Here's the drawing with two shaded views (mm, measured from the low corner). I have some questions. Round coordinates to 2 decimals unless told otherwise and drop trailing zeros. Loops run counter-clockwise (first coordinate to the right, second up) from the corner with the lowest first, then second, coordinate; pieces in that order, holes last.
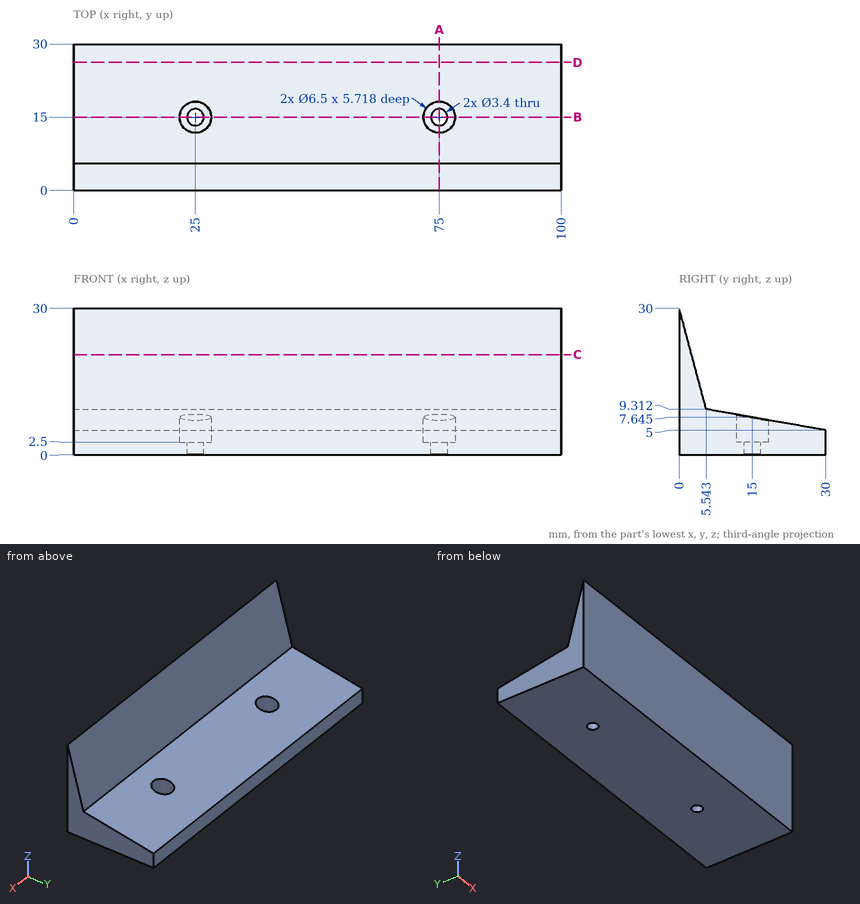
(1) If we section it at B-B, the plane y = 15: State how many separate pieces and enclosed holes the cut face has.
Worked answers:
separate pieces: 3
enclosed holes: 0
(2) If we section it at C-C, the plane z = 20.5: List the corners of the cut face in (x, y) for me (1 decimal).
Worked answers:
outline: (0, 0) - (100, 0) - (100, 2.5) - (0, 2.5) - close
(3) If we section it at D-D, the plane y = 26.25: List the corners of the cut face in (x, z) for me.
Worked answers:
outline: (0, 0) - (100, 0) - (100, 5.66) - (0, 5.66) - close
(4) If we section it at A-A, the plane x = 75: List the corners of the cut face in (y, z) for me.
Worked answers:
outline: (0, 0) - (13.3, 0) - (13.3, 2.5) - (11.75, 2.5) - (11.75, 8.22) - (5.54, 9.31) - (0, 30) - close; (16.7, 0) - (30, 0) - (30, 5) - (18.25, 7.07) - (18.25, 2.5) - (16.7, 2.5) - close
(5) Will these pins go through, and if not, where does the flat tip stop? P1, Ø10, axis at x = 51.5, y = 19, coming from the -Z side; P2, Ø7, axis at x = 24.5, y = 16.5, coming from the +Z side; P3, Ø6, axis at x = 75, y = 15, coming from the +Z side; P4, Ø3, axis at y = 4, z = 23, coming from the -X side.
Worked answers:
P1: stops at z = 0
P2: stops at z = 7.78
P3: stops at z = 2.5
P4: passes through
(6) If I drill on line 1 (Y direction, x = 75, z = 0.85); line 2 (Y direction, x = 25, z = 3.7); line 3 (Z direction, x = 62.5, y = 21.5), over which ranges is the centre line in solid material (lowest first)?
Worked answers:
line 1: y = 0 to 13.3, 16.7 to 30
line 2: y = 0 to 11.75, 18.25 to 30
line 3: z = 0 to 6.5
